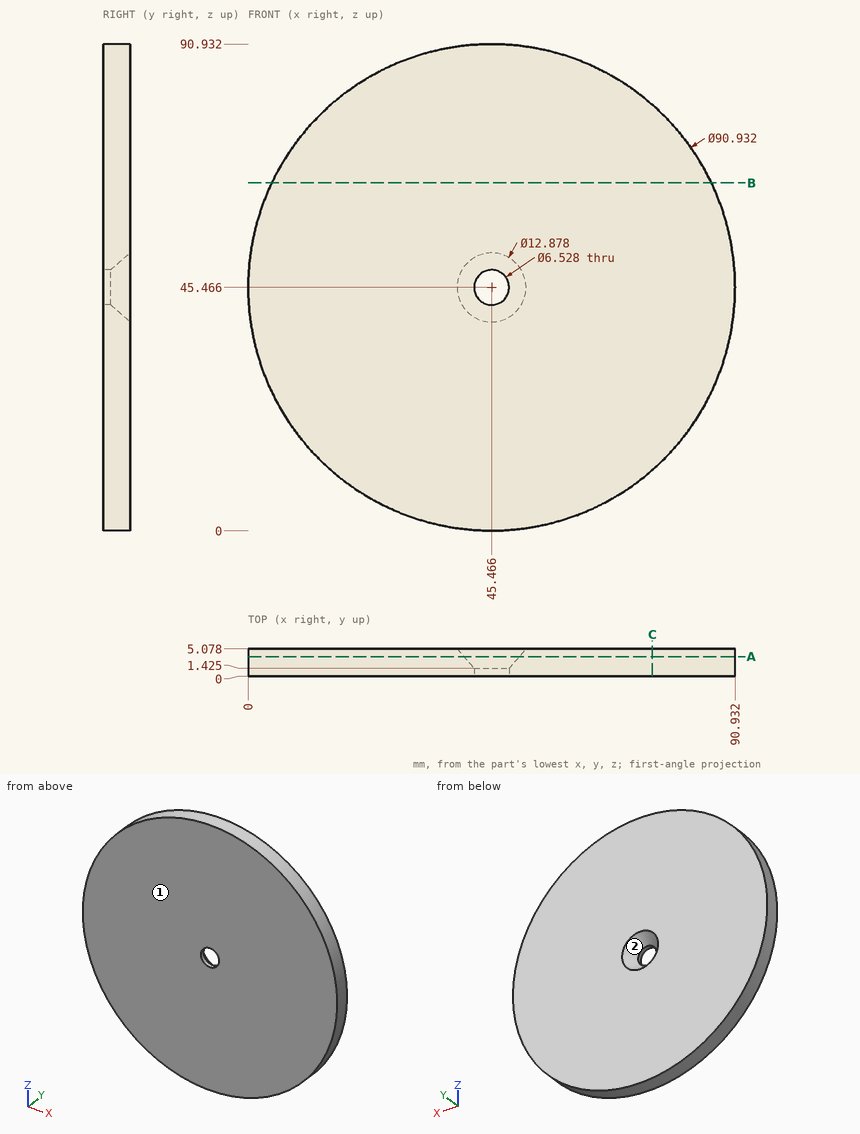
Answer from the drawing. Dimensions are ordinates in mm from the lowest x, y and z of the part. Round coordinates to 2 decimals unless told otherwise and drop trailing zeros. Write each loop counter-clockwise with the first axis right and the second up, starting at its lowest first coordinate (ties: lowest second). Pieces come first, ordered by that corner, then holes. Notation, with made-up numbers: (85.25, -36) - (143.25, -36) arc R18 ccw to (143.25, -2) - close; hole circle Ø9 at (-5.5, 77.25). An arc over 180 degrees is marked (long way). One line per item, written item: value.
Q1. For a pull along Z with two mould halves and no side action, classify the marked faces 1 and 2 as pulls with the +Z half, pulls with the -Z half, needs draft (parallel to the pull), parting line crosses it, or undercut.
The answers:
face 1: needs draft
face 2: undercut
Q2. Find section A-A (y = 3.6). Determine the outline of the cut face in (x, z) (1 decimal), and give its area (3 significant figures).
The answers:
outline: circle Ø90.9 at (45.5, 45.5); hole circle Ø10.3 at (45.5, 45.5)
area: 6,410 mm2
Q3. Find section B-B (z = 65). Determine the outline of the cut face in (x, y), and give its area (3 significant figures).
The answers:
outline: (4.41, 0) - (86.52, 0) - (86.52, 5.08) - (4.41, 5.08) - close
area: 417 mm2
Q4. Straight lines are drawn through the part: line 1 (Z direction, x = 48, y = 3.2); line 2 (Z direction, x = 47.5, y = 3.2) (1 decimal); line 3 (Z direction, x = 35, y = 4.15). For each, find the intervals that lie inside material, in ascending order. Write a range as from..to.
The answers:
line 1: z = 0.07..41.38, 49.55..90.86
line 2: z = 0..41.1, 49.8..90.9
line 3: z = 1.22..89.71
Q5. Each of these flat-tipped pins is pushed along its axis until it touches: P1, Ø3, axis at x = 62.5, y = 2, coming from the -Z side; P2, Ø3, axis at x = 33.5, y = 4.5, coming from the +Z side. Where does it stop, or does it pass through?
The answers:
P1: stops at z = 2.74
P2: stops at z = 89.71
Q6. Find section C-C (x = 75.5). Determine the outline of the cut face in (y, z).
The answers:
outline: (0, 11.33) - (5.08, 11.33) - (5.08, 79.6) - (0, 79.6) - close
